```python
from build123d import *
from OCP.BRepFilletAPI import BRepFilletAPI_MakeChamfer

# Parameters (mm, degrees)
SKETCH5_R            = 250
BOSS_EXTRUDE4_DEPTH  = 100
SKETCH6_W            = 200
SKETCH6_H            = 100
SKETCH6_W_2          = 100
SKETCH6_H_2          = 200
BOSS_EXTRUDE5_DEPTH  = 100
BOSS_EXTRUDE6_DEPTH  = 15
BOSS_EXTRUDE7_DEPTH  = 10
BOSS_EXTRUDE8_DEPTH  = 10
SKETCH18_R           = 15
CUT_EXTRUDE2_DEPTH   = 587.024743505
BOSS_EXTRUDE9_DEPTH  = 10
BOSS_EXTRUDE10_START = -10
BOSS_EXTRUDE10_DEPTH = 10
BOSS_EXTRUDE11_DEPTH = 10
BOSS_EXTRUDE12_DEPTH = 10
SKETCH24_R           = 200
BOSS_EXTRUDE13_DEPTH = 25
SKETCH25_R           = 25
BOSS_EXTRUDE14_DEPTH = 50
BOSS_EXTRUDE15_DEPTH = 40
CHAMFER1_SIZE        = 10
CHAMFER1_SIZE2       = 17.320508076
CHAMFER2_SIZE        = 10


with BuildPart() as part:
    # Sketch5 → Boss-Extrude4 (new body)
    with BuildSketch(Plane(origin=(0, 0, 0), x_dir=(1, 0, 0), z_dir=(0, 1, 0))):
        with Locations(Location((0, 0, 0), (0, 0, 270))):
            Circle(SKETCH5_R)
    extrude(amount=BOSS_EXTRUDE4_DEPTH)

    # Sketch6 → Boss-Extrude5 (add)
    with BuildSketch(Plane(origin=(0, 100, 0), x_dir=(1, 0, 0), z_dir=(0, 1, 0))):
        with Locations((0, -250)):
            Rectangle(SKETCH6_W, SKETCH6_H)
        with Locations((0, 250)):
            Rectangle(SKETCH6_W, SKETCH6_H)
        with Locations((250, 0)):
            Rectangle(SKETCH6_W_2, SKETCH6_H_2)
        with Locations((-250, 0)):
            Rectangle(SKETCH6_W_2, SKETCH6_H_2)
    extrude(amount=-BOSS_EXTRUDE5_DEPTH)

    # Sketch10 → Boss-Extrude6 (add)
    with BuildSketch(Plane.XZ):
        with BuildLine():
            Line((-100, 300), (-100, 400))
            ThreePointArc((-100, 400), (-97.071067812, 407.071067812), (-90, 410))
            Line((-90, 410), (90, 410))
            ThreePointArc((90, 410), (97.071067812, 407.071067812), (100, 400))
            Line((100, 400), (100, 300))
            Line((100, 300), (-100, 300))
        make_face()
        with BuildLine():
            Line((100, -310), (100, -400))
            ThreePointArc((100, -400), (97.071067812, -407.071067812), (90, -410))
            Line((90, -410), (-90, -410))
            ThreePointArc((-90, -410), (-97.071067812, -407.071067812), (-100, -400))
            Line((-100, -400), (-100, -300))
            Line((-100, -300), (90, -300))
            Line((90, -300), (100, -300))
            Line((100, -300), (100, -310))
        make_face()
        with BuildLine():
            Line((-300, -100), (-400, -100))
            ThreePointArc((-400, -100), (-407.071067812, -97.071067812), (-410, -90))
            Line((-410, -90), (-410, 90))
            ThreePointArc((-410, 90), (-407.071067812, 97.071067812), (-400, 100))
            Line((-400, 100), (-300, 100))
            Line((-300, 100), (-300, -100))
        make_face()
        with BuildLine():
            Line((300, -100), (400, -100))
            ThreePointArc((400, -100), (407.071067812, -97.071067812), (410, -90))
            Line((410, -90), (410, 90))
            ThreePointArc((410, 90), (407.071067812, 97.071067812), (400, 100))
            Line((400, 100), (300, 100))
            Line((300, 100), (300, -100))
        make_face()
    extrude(amount=-BOSS_EXTRUDE6_DEPTH)

    # Sketch12 → Boss-Extrude7 (add)
    with BuildSketch(Plane(origin=(100, 0, 0), x_dir=(0, 0, -1), z_dir=(1, 0, 0))):
        Polygon((-400, 15), (-400, 45), (-368.245735195, 100), (-300, 100), (-300, 15), align=None)
    extrude(amount=-BOSS_EXTRUDE7_DEPTH)

    # Sketch13 → Boss-Extrude8 (add)
    with BuildSketch(Plane.ZY.offset(100)):
        Polygon((300, 100), (300, 15), (400, 15), (400, 45), (368.245735195, 100), align=None)
    extrude(amount=-BOSS_EXTRUDE8_DEPTH)

    # Sketch18 → Cut-Extrude2 (cut, through all)
    with BuildSketch(Plane(origin=(0, 15, 0), x_dir=(1, 0, 0), z_dir=(0, 1, 0))):
        with Locations(Location((-50, -350, 0), (0, 0, 270))):
            Circle(SKETCH18_R)
        with Locations(Location((50, -350, 0), (0, 0, 270))):
            Circle(SKETCH18_R)
        with Locations(Location((-350, 50, 0), (0, 0, 270))):
            Circle(SKETCH18_R)
        with Locations(Location((-350, -50, 0), (0, 0, 270))):
            Circle(SKETCH18_R)
        with Locations(Location((-50, 350, 0), (0, 0, 270))):
            Circle(SKETCH18_R)
        with Locations(Location((50, 350, 0), (0, 0, 270))):
            Circle(SKETCH18_R)
        with Locations(Location((350, 50, 0), (0, 0, 270))):
            Circle(SKETCH18_R)
        with Locations(Location((350, -50, 0), (0, 0, 270))):
            Circle(SKETCH18_R)
    extrude(amount=-CUT_EXTRUDE2_DEPTH, mode=Mode.SUBTRACT)

    # Sketch19 → Boss-Extrude9 (add)
    with BuildSketch(Plane.XY.offset(100)):
        with BuildLine():
            Line((-400, 15), (-400, 45))
            Line((-400, 45), (-371.132486541, 95))
            ThreePointArc((-371.132486541, 95), (-367.472232503, 98.660254038), (-362.472232503, 100))
            Line((-362.472232503, 100), (-300, 100))
            Line((-300, 100), (-300, 15))
            Line((-300, 15), (-400, 15))
        make_face()
        with BuildLine():
            Line((400, 15), (400, 45))
            Line((400, 45), (371.132486541, 95))
            ThreePointArc((371.132486541, 95), (367.472232503, 98.660254038), (362.472232503, 100))
            Line((362.472232503, 100), (300, 100))
            Line((300, 100), (300, 15))
            Line((300, 15), (400, 15))
        make_face()
    extrude(amount=-BOSS_EXTRUDE9_DEPTH)

    # Sketch20 → Boss-Extrude10 (add)
    with BuildSketch(Plane(origin=(0, 0, -100), x_dir=(-1, 0, 0), z_dir=(0, 0, -1)).offset(BOSS_EXTRUDE10_START)):
        with BuildLine():
            Line((-400, 15), (-400, 45))
            Line((-400, 45), (-371.132486541, 95))
            ThreePointArc((-371.132486541, 95), (-367.472232503, 98.660254038), (-362.472232503, 100))
            Line((-362.472232503, 100), (-300, 100))
            Line((-300, 100), (-300, 15))
            Line((-300, 15), (-400, 15))
        make_face()
        with BuildLine():
            Line((400, 15), (400, 45))
            Line((400, 45), (371.132486541, 95))
            ThreePointArc((371.132486541, 95), (367.472232503, 98.660254038), (362.472232503, 100))
            Line((362.472232503, 100), (300, 100))
            Line((300, 100), (300, 15))
            Line((300, 15), (400, 15))
        make_face()
    extrude(amount=BOSS_EXTRUDE10_DEPTH)

    # Sketch22 → Boss-Extrude11 (add)
    with BuildSketch(Plane(origin=(100, 0, 0), x_dir=(0, 0, -1), z_dir=(1, 0, 0))):
        Polygon((400, 15), (400, 45), (368.245735195, 100), (300, 100), (300, 15), align=None)
    extrude(amount=-BOSS_EXTRUDE11_DEPTH)

    # Sketch23 → Boss-Extrude12 (add)
    with BuildSketch(Plane.ZY.offset(100)):
        with BuildLine():
            Line((-400, 15), (-400, 45))
            Line((-400, 45), (-371.132486541, 95))
            ThreePointArc((-371.132486541, 95), (-367.472232503, 98.660254038), (-362.472232503, 100))
            Line((-362.472232503, 100), (-300, 100))
            Line((-300, 100), (-300, 15))
            Line((-300, 15), (-400, 15))
        make_face()
    extrude(amount=-BOSS_EXTRUDE12_DEPTH)

    # Sketch24 → Boss-Extrude13 (add)
    with BuildSketch(Plane(origin=(0, 100, 0), x_dir=(1, 0, 0), z_dir=(0, 1, 0))):
        with Locations(Location((0, 0, 0), (0, 0, 270))):
            Circle(SKETCH24_R)
    extrude(amount=BOSS_EXTRUDE13_DEPTH)

    # Sketch25 → Boss-Extrude14 (add)
    with BuildSketch(Plane(origin=(0, 125, 0), x_dir=(1, 0, 0), z_dir=(0, 1, 0))):
        with Locations(Location((0, 0, 0), (0, 0, 270))):
            Circle(SKETCH25_R)
    extrude(amount=BOSS_EXTRUDE14_DEPTH)

    # Sketch27 → Boss-Extrude15 (add)
    with BuildSketch(Plane.XZ):
        with BuildLine():
            Line((-256.173769149, 100), (-229.128784748, 100))
            ThreePointArc((-229.128784748, 100), (-176.776695297, 176.776695297), (-100, 229.128784748))
            Line((-100, 229.128784748), (-100, 256.173769149))
            ThreePointArc((-100, 256.173769149), (-194.454364826, 194.454364826), (-256.173769149, 100))
        make_face()
        with BuildLine():
            Line((100, 229.128784748), (100, 256.173769149))
            ThreePointArc((100, 256.173769149), (194.454364826, 194.454364826), (256.173769149, 100))
            Line((256.173769149, 100), (229.128784748, 100))
            ThreePointArc((229.128784748, 100), (176.776695297, 176.776695297), (100, 229.128784748))
        make_face()
        with BuildLine():
            Line((100, -256.173769149), (100, -229.128784748))
            ThreePointArc((100, -229.128784748), (176.776695297, -176.776695297), (229.128784748, -100))
            Line((229.128784748, -100), (256.173769149, -100))
            ThreePointArc((256.173769149, -100), (194.454364826, -194.454364826), (100, -256.173769149))
        make_face()
        with BuildLine():
            Line((-100, -256.173769149), (-100, -229.128784748))
            ThreePointArc((-100, -229.128784748), (-176.776695297, -176.776695297), (-229.128784748, -100))
            Line((-229.128784748, -100), (-256.173769149, -100))
            ThreePointArc((-256.173769149, -100), (-194.454364826, -194.454364826), (-100, -256.173769149))
        make_face()
    extrude(amount=-BOSS_EXTRUDE15_DEPTH)

    # Chamfer1: one chamfer whose edges measure the first distance from different faces: ONE call of the kernel's chamfer builder (chamfer() names one face for all edges)
    chamfer1_edges_1 = [part.edges().sort_by_distance(p)[0] for p in [
        (194.454364826, 40, -194.454364826),
    ]]
    chamfer1_side_1 = [part.faces().sort_by_distance(p)[0] for p in [
        (181.097571565, 40, -181.097571565),
    ]]
    chamfer1_edges_2 = [part.edges().sort_by_distance(p)[0] for p in [
        (194.454364826, 40, 194.454364826),
    ]]
    chamfer1_side_2 = [part.faces().sort_by_distance(p)[0] for p in [
        (181.097571565, 40, 181.097571565),
    ]]
    chamfer1_edges_3 = [part.edges().sort_by_distance(p)[0] for p in [
        (-194.454364826, 40, 194.454364826),
    ]]
    chamfer1_side_3 = [part.faces().sort_by_distance(p)[0] for p in [
        (-181.097571565, 40, 181.097571565),
    ]]
    chamfer1_edges_4 = [part.edges().sort_by_distance(p)[0] for p in [
        (-194.454364826, 40, -194.454364826),
    ]]
    chamfer1_side_4 = [part.faces().sort_by_distance(p)[0] for p in [
        (-181.097571565, 40, -181.097571565),
    ]]
    chamfer1 = BRepFilletAPI_MakeChamfer(part.part.solid().wrapped)
    for e in chamfer1_edges_1:
        chamfer1.Add(CHAMFER1_SIZE, CHAMFER1_SIZE2, e.wrapped, chamfer1_side_1[0].wrapped)  # the first distance lies on this face
    for e in chamfer1_edges_2:
        chamfer1.Add(CHAMFER1_SIZE, CHAMFER1_SIZE2, e.wrapped, chamfer1_side_2[0].wrapped)  # the first distance lies on this face
    for e in chamfer1_edges_3:
        chamfer1.Add(CHAMFER1_SIZE, CHAMFER1_SIZE2, e.wrapped, chamfer1_side_3[0].wrapped)  # the first distance lies on this face
    for e in chamfer1_edges_4:
        chamfer1.Add(CHAMFER1_SIZE, CHAMFER1_SIZE2, e.wrapped, chamfer1_side_4[0].wrapped)  # the first distance lies on this face
    add(Compound.cast(chamfer1.Shape()), mode=Mode.REPLACE)

    # Chamfer2
    chamfer2_edges = [part.edges().sort_by_distance(p)[0] for p in [
        (0, 125, -200),
    ]]
    chamfer(chamfer2_edges, length=CHAMFER2_SIZE)


solid = part.part
```
Check sheet for the modelled part. Datum: model origin and axes. Units: mm. A direction names the side the tool comes from. Round coordinates to 2 decimals unless told otherwise and drop trailing zeros. Order: outer loops, then holes, each group sorted by start corner. A loop starts at its lowest first (then second) coordinate and runs counter-clockwise, first axis right, second up. Notation, with made-up numbers: (57.25, 51) - (91.25, 51) arc R20 cw to (91.25, 74) - close; hole circle Ø7 at (85, 89). An arc over 180 degrees is marked (long way). Answer as CSV lines item,"result". Start each with the question number.
1) Draft check along X on faces 5 (the face through (-385.77, 69.65, -94.93)), 6 (the face through (364.872, 7.605, 48.047)), 7 (the face through (178, 40, -178)), 8 (the face through (100, 51, -313)). Enter one of: +X half, -X half, draft (parallel to the pull), parting line (faces both ways), or undercut.
2) Depth check by flat-ended pin: pin 1 (18 mm diameter, centred on x = 50, z = -350, fed in from +Y); pin 2 (3 mm diameter, centred on x = 157, z = 4, fed in from +Y); pin 3 (3 mm diameter, centred on y = 27.5, z = 95, fed in from +X); pin 4 (4 mm diameter, centred on x = -192, y = 30.5, fed in from +Z). Enter the tip coordinate at first touch or a pass-through.
3) Tool access check on faces 1 (the face through (-178, 40, 178)), 2 (the face through (7.509, 149.65, 23.846)), 3 (the face through (-90, 58, -349)), 4 (the face through (300, 58, 1)). Record the directions out of +Z, -Z, +X, -X, +Y, -Y that give a thin tool (end or side, any length) a straight path to the whole face; none if there is none.
4) Section check D-D (z = 0). Record the cut outline in (x, y).
5) Scan lines: probe 1 along X at (y, z) = (8.75, -50); probe 2 along X at (y, z) = (6.5, 350); probe 3 along Z at (x, y) = (366, 83). Record each from-to range of solid material in increasing order.
6) Section check A-A (z = -350). Record the cut outline in (x, y), then the cut area to 3 significant figures.
7) Section check B-B (x = 350). Record the cut outline in (y, z).
Determined:
1,face 5,"-X half"
1,face 6,"undercut"
1,face 7,"draft"
1,face 8,"+X half"
2,pin 1,"through"
2,pin 2,"y = 125"
2,pin 3,"x = 400"
2,pin 4,"z = 193.1"
3,face 1,"+Z, -X, +Y"
3,face 2,"+Y"
3,face 3,"-Z, +Y"
3,face 4,"+X, +Y"
4,outline,"(-410, 0) - (410, 0) - (410, 15) - (300, 15) - (300, 100) - (200, 100) - (200, 115) - (190, 125) - (25, 125) - (25, 175) - (-25, 175) - (-25, 125) - (-190, 125) - (-200, 115) - (-200, 100) - (-300, 100) - (-300, 15) - (-410, 15) - close"
5,probe 1,"-410 to -365, -335 to 335, 365 to 410"
5,probe 2,"-100 to -65, -35 to 35, 65 to 100"
5,probe 3,"-100 to -90, 90 to 100"
6,outline,"(-100, 0) - (-65, 0) - (-65, 15) - (-90, 15) - (-90, 100) - (-100, 100) - close; (-35, 0) - (35, 0) - (35, 15) - (-35, 15) - close; (65, 0) - (100, 0) - (100, 100) - (90, 100) - (90, 15) - (65, 15) - close"
6,area,"3,800 mm^2"
7,outline,"(0, -100) - (100, -100) - (100, -90) - (15, -90) - (15, -65) - (0, -65) - close; (0, -35) - (15, -35) - (15, 35) - (0, 35) - close; (0, 65) - (15, 65) - (15, 90) - (100, 90) - (100, 100) - (0, 100) - close"
